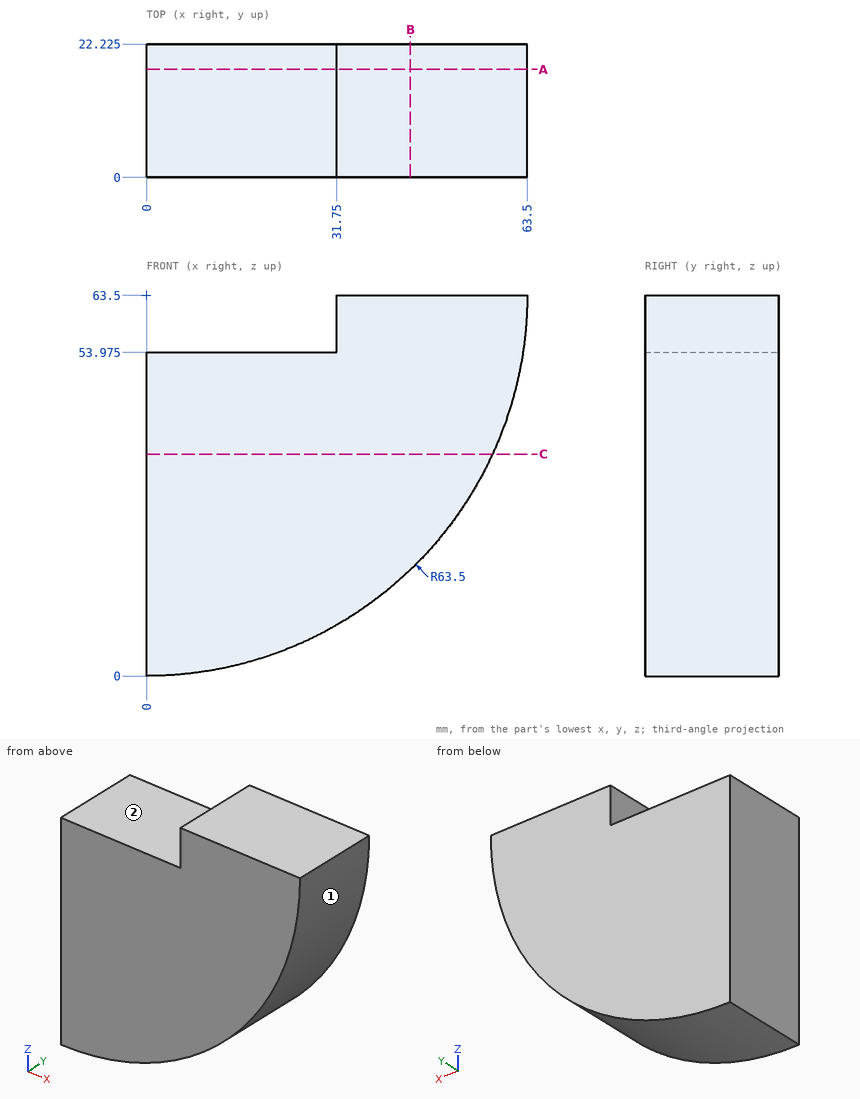
Answer from the drawing. Dimensions are ordinates in mm from the lowest x, y and z of the part. A direction names the side the tool comes from. Give positions to 0.01 mm unless a question says otherwise; leave off trailing zeros. Loops run counter-clockwise (first coordinate to the right, second up) from the corner with the lowest first, then second, coordinate; pieces in that order, holes last. Notation, with made-up numbers: (-10.5, -33) - (23.5, -33) arc R14 ccw to (23.5, -12) - close; hole circle Ø5 at (-10.5, 5). An arc over 180 degrees is marked (long way). Answer as CSV lines item,"result". Start each with the question number.
Item 1: A cutting plane is placed at B-B on x = 44. Determine the outline of the cut face in (y, z) (3 decimals).
Item 2: For the marked faces 1 and 2, determine the directions among +Z, -Z, +X, -X, +Y, -Y from which every point of the face is accessible in a straight line to the end or side of a thin tool.
Item 3: Each of these flat-tipped pins is pushed along its axis until it touches: pin 1 (10 mm diameter, centred on y = 16, z = 7, fed in from +X); pin 2 (8 mm diameter, centred on x = 6.5, y = 19, fed in from -Z); pin 3 (5 mm diameter, centred on y = 15, z = 57, fed in from -X); pin 4 (6 mm diameter, centred on x = 29, y = 6, fed in from +Z). Where does it stop, or does it pass through?
Item 4: Find the intervals of material crossed by line 1 (X direction, y = 18.75, z = 57); line 2 (Z direction, x = 36.5, y = 3.75); line 3 (Z direction, x = 36, y = 10.75), in increasing order. Write a range as from..to.
Item 5: A cutting plane is placed at C-C on z = 37. Determine the outline of the cut face in (x, y) (3 decimals), then the cut area to 3 significant figures.
Item 6: A cutting plane is placed at A-A on y = 18. Determine the outline of the cut face in (x, z) (3 decimals).
Found:
1,outline,"(0, 17.715) - (22.225, 17.715) - (22.225, 63.5) - (0, 63.5) - close"
2,face 1,"-Z, +X, +Y, -Y"
2,face 2,"+Z, -X, +Y, -Y"
3,pin 1,"stops at x = 37.15"
3,pin 2,"stops at z = 0.05"
3,pin 3,"stops at x = 31.75"
3,pin 4,"stops at z = 63.5"
4,line 1,"x = 31.75..63.17"
4,line 2,"z = 11.54..63.5"
4,line 3,"z = 11.19..63.5"
5,outline,"(0, 0) - (57.706, 0) - (57.706, 22.225) - (0, 22.225) - close"
5,area,"1,280 mm^2"
6,outline,"(0, 0) arc R63.5 ccw to (63.5, 63.5) - (31.75, 63.5) - (31.75, 53.975) - (0, 53.975) - close"
